For this review, take the finished solid that the model builds, in its own axes (mm). Give positions to 0.01 mm unless a question says otherwise; leave off trailing zeros. Loops run counter-clockwise (first coordinate to the right, second up) from the corner with the lowest first, then second, coordinate; pieces in that order, holes last. Notation, with made-up numbers: (62, 64) - (107, 64) arc R32 ccw to (107, 94) - close; hole circle Ø9 at (44.5, 66.25). An arc over 180 degrees is marked (long way). Use CSV: the item, a comma, the result in double quotes. Start each with the question number.
1. Wall thickness on line 1 (Y direction, x = 5.08, z = 160); line 2 (Z direction, x = -3, y = 11.5) (3 decimals); line 3 (Z direction, x = 2.5, y = 2.5) (3 decimals): over which ranges is each line inside the solid? List them lowest first.
2. Take a section at B-B on z = 195. Give the boundary of the cut face in (x, y), plus the area to 3 significant figures.
3. Take a section at A-A on x = 5.08. Give the boundary of the cut face in (y, z) (3 decimals), plus the area to 3 significant figures.
4. For pin 1 (4 mm diameter, centred on x = 9, z = 90.5, fed in from +Y); pin 2 (1.5 mm diameter, centred on x = 3.5, z = 184, fed in from -Y); pin 3 (11 mm diameter, centred on x = 3, z = 9.5, fed in from -Y), all flat-tipped, find the tip position at first contact; note any pin that passes through.
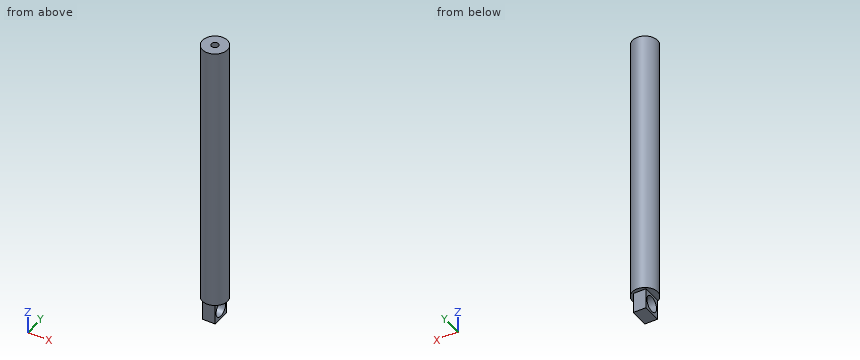
Autodesk Inventor part; units mm, degrees
ref_plane "YZ Plane" through (0, 0, 0) normal (1, 0, 0) x (0, 1, 0)
ref_plane "XZ Plane" through (0, 0, 0) normal (0, 1, 0) x (-1, 0, 0)
ref_plane "XY Plane" through (0, 0, 0) normal (0, 0, 1) x (1, 0, 0)
sketch "Sketch1" plane through (0, 0, 0) normal (0, 0, 1) x (1, 0, 0)
  line L0 (0, 0) -> (10.16, 0)
  line L1 (10.16, 0) -> (10.16, 15.24)
  line L2 (10.16, 15.24) -> (0, 15.24)
  line L3 (0, 15.24) -> (0, 0)
  dimension "d0" = 10.16
  dimension "d1" = 15.24
extrude "Extrusion1" add sketch "Sketch1" along normal blind 16.51
sketch "Sketch2" plane through (10.16, 0, 0) normal (1, 0, 0) x (0, 0, -1)
  circle A0 centre (-8.255, 7.62) radius 6.35
  line L0 (0, 15.24) -> (-16.51, 15.24)
  point P0 (0, 0)
  dimension "d4" = 12.7
  dimension "d5" = 7.62
extrude "Extrusion2" cut sketch "Sketch2" against normal blind 16.51
sketch "Sketch3" plane through (0, 0, 16.51) normal (0, 0, 1) x (1, 0, 0)
  circle A0 centre (5.08, 8.152) radius 10.16
  point P0 (0, 0)
  dimension "d8" = 20.32
extrude "Extrusion3" add sketch "Sketch3" along normal blind 219.075
sketch "Sketch5" plane through (5.08, 8.152, 235.585) normal (0, 0, 1) x (1, 0, 0)
  circle A0 centre (0, 0) radius 2.921
  point P0 (-5.08, -8.152)
  dimension "d13" = 5.842
extrude "Extrusion5" cut sketch "Sketch5" against normal blind 152.4
properties part number "SolenoidCase"
Check result:
1,line 1,"y = -2.01 to 5.23, 11.07 to 18.31"
1,line 2,"z = 16.51 to 235.585"
1,line 3,"z = 0 to 4.499, 12.011 to 235.585"
2,outline,"circle Ø20.32 at (5.08, 8.15); hole circle Ø5.84 at (5.08, 8.15)"
2,area,"297 mm²"
3,outline,"(-2.008, 16.51) - (0, 16.51) - (0, 0) - (15.24, 0) - (15.24, 16.51) - (18.312, 16.51) - (18.312, 235.585) - (11.073, 235.585) - (11.073, 83.185) - (5.231, 83.185) - (5.231, 235.585) - (-2.008, 235.585) - close; hole circle Ø12.7 at (7.62, 8.255)"
3,area,"3,690 mm²"
4,pin 1,"stops at y = 18.13"
4,pin 2,"stops at y = -1.97"
4,pin 3,"stops at y = 0"
